Source: CAD feature listing. Evaluate the final solid. Frame: model axes, mm. Face numbers are marked on the shaded views. A direction names the side the tool comes from. Give positions to 0.01 mm unless a question says otherwise; leave off trailing zeros. Order: outer loops, then holes, each group sorted by start corner. A loop starts at its lowest first (then second) coordinate and runs counter-clockwise, first axis right, second up. Notation, with made-up numbers: M 61.5,18 L 96.5,18 A18 ccw 96.5,38 Z; hole C -7,23 d1. An arc over 180 degrees is marked long. Return JSON: item names as keys, results as strings.
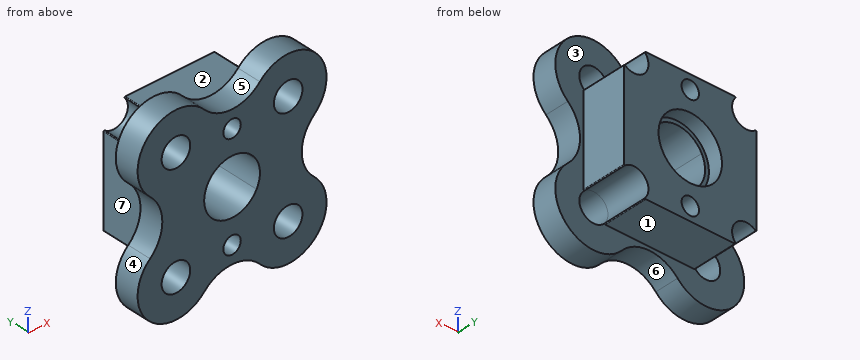
from build123d import *
from build123d.topology import SkipClean

# Parameters (mm, degrees)
SKETCH1_R               = 1.25
BOSS_EXTRUDE1_DEPTH     = 3.5
SKETCH3_R               = 2.05
CUT_EXTRUDE3_DEPTH      = 20.479604719
BOSS_EXTRUDE2_START     = 6.5
SKETCH6_R               = 1.25
BOSS_EXTRUDE2_DEPTH     = 6.5
CUT_EXTRUDE8_DEPTH      = 22.614925399
CUT_EXTRUDE7_DEPTH      = 22.614925399
CUT_EXTRUDE7_DEPTH_BACK = 22.614925399
SKETCH9_R               = 4
SKETCH11_R              = 4.55
CUT_EXTRUDE9_DEPTH      = 2.1
FILLET5_R               = 0.1


with BuildPart() as part:
    # Sketch1 → Boss-Extrude1 (new body)
    with BuildSketch(Plane(origin=(0, 0, 0), x_dir=(1, 0, 0), z_dir=(0, 1, 0))):
        with BuildLine():
            ThreePointArc((3.988860539, -11.759062722), (11.939087297, -11.939087297), (11.759062722, -3.988860539))
            ThreePointArc((11.759062722, -3.988860539), (10, 0), (11.759062722, 3.988860539))
            ThreePointArc((11.759062722, 3.988860539), (11.939087297, 11.939087297), (3.988860539, 11.759062722))
            ThreePointArc((3.988860539, 11.759062722), (0, 10), (-3.988860539, 11.759062722))
            ThreePointArc((-3.988860539, 11.759062722), (-11.939087297, 11.939087297), (-11.759062722, 3.988860539))
            ThreePointArc((-11.759062722, 3.988860539), (-10, 0), (-11.759062722, -3.988860539))
            ThreePointArc((-11.759062722, -3.988860539), (-11.939087297, -11.939087297), (-3.988860539, -11.759062722))
            ThreePointArc((-3.988860539, -11.759062722), (0, -10), (3.988860539, -11.759062722))
        make_face()
        with Locations(Location((0, -7.5, 0), (0, 0, 270))):
            Circle(SKETCH1_R, mode=Mode.SUBTRACT)
        with Locations(Location((0, 7.5, 0), (0, 0, 90))):
            Circle(SKETCH1_R, mode=Mode.SUBTRACT)
    extrude(amount=BOSS_EXTRUDE1_DEPTH)

    # Sketch3 → Cut-Extrude3 (cut, through all)
    with BuildSketch(Plane(origin=(0, 3.5, 0), x_dir=(1, 0, 0), z_dir=(0, 1, 0))):
        with Locations(Location((-8.05, 8.05, 0), (0, 0, 270))):
            Circle(SKETCH3_R)
        with Locations(Location((8.05, 8.05, 0), (0, 0, 270))):
            Circle(SKETCH3_R)
        with Locations(Location((8.05, -8.05, 0), (0, 0, 270))):
            Circle(SKETCH3_R)
        with Locations(Location((-8.05, -8.05, 0), (0, 0, 270))):
            Circle(SKETCH3_R)
    extrude(amount=-CUT_EXTRUDE3_DEPTH, mode=Mode.SUBTRACT)

    # Sketch6 → Boss-Extrude2 (add)
    with SkipClean():  # the faces are left unmerged after this step: merging them gives an invalid solid
        with BuildSketch(Plane(origin=(0, 3.5, 0), x_dir=(1, 0, 0), z_dir=(0, 1, 0)).offset(BOSS_EXTRUDE2_START)):
            with BuildLine():
                Line((6.600862325, 9.5), (-6.600862325, 9.5))
                ThreePointArc((-6.600862325, 9.5), (-6.600431099, 6.600431099), (-9.5, 6.600862325))
                Line((-9.5, 6.600862325), (-9.5, -6.600862325))
                ThreePointArc((-9.5, -6.600862325), (-6.600431099, -6.600431099), (-6.600862325, -9.5))
                Line((-6.600862325, -9.5), (6.600862325, -9.5))
                ThreePointArc((6.600862325, -9.5), (6.600431099, -6.600431099), (9.5, -6.600862325))
                Line((9.5, -6.600862325), (9.5, 6.600862325))
                ThreePointArc((9.5, 6.600862325), (6.600431099, 6.600431099), (6.600862325, 9.5))
            make_face()
            with Locations(Location((0, -7.5, 0), (0, 0, 270))):
                Circle(SKETCH6_R, mode=Mode.SUBTRACT)
            with Locations(Location((0, 7.5, 0), (0, 0, 90))):
                Circle(SKETCH6_R, mode=Mode.SUBTRACT)
        extrude(amount=-BOSS_EXTRUDE2_DEPTH)

    # Sketch10 → Cut-Extrude8 (cut, through all)
    with SkipClean():  # the faces are left unmerged after this step: merging them gives an invalid solid
        with BuildSketch(Plane(origin=(0, 10, 0), x_dir=(1, 0, 0), z_dir=(0, 1, 0))):
            with BuildLine():
                Line((-3.519943181, 1.9), (-3.519943181, -1.9))
                ThreePointArc((-3.519943181, -1.9), (0, -4), (3.519943181, -1.9))
                Line((3.519943181, -1.9), (3.519943181, 1.9))
                ThreePointArc((3.519943181, 1.9), (0, 4), (-3.519943181, 1.9))
            make_face()
        extrude(amount=-CUT_EXTRUDE8_DEPTH, mode=Mode.SUBTRACT)

    # Sketch9 → Cut-Extrude7 (cut, two sides: drawn at the far end of the back side and taken through both)
    with SkipClean():  # the faces are left unmerged after this step: merging them gives an invalid solid
        with BuildSketch(Plane(origin=(0, 10, 0), x_dir=(1, 0, 0), z_dir=(0, 1, 0)).offset(-CUT_EXTRUDE7_DEPTH_BACK)):
            with Locations(Location((0, 0, 0), (0, 0, 90))):
                Circle(SKETCH9_R)
        extrude(amount=CUT_EXTRUDE7_DEPTH + CUT_EXTRUDE7_DEPTH_BACK, mode=Mode.SUBTRACT)

    # Sketch11 → Cut-Extrude9 (cut)
    with SkipClean():  # the faces are left unmerged after this step: merging them gives an invalid solid
        with BuildSketch(Plane(origin=(0, 10, 0), x_dir=(1, 0, 0), z_dir=(0, 1, 0))):
            with Locations(Location((0, 0, 0), (0, 0, 270))):
                Circle(SKETCH11_R)
        extrude(amount=-CUT_EXTRUDE9_DEPTH, mode=Mode.SUBTRACT)

    # Fillet5
    fillet5_edges = [part.edges().sort_by_distance(p)[0] for p in [
        (9.5, 6.75, -6.600862325),
        (6.600862325, 6.75, -9.5),
        (9.5, 6.75, 6.600862325),
        (6.600862325, 6.75, 9.5),
        (-6.600862325, 6.75, 9.5),
        (-9.5, 6.75, 6.600862325),
        (-9.5, 6.75, -6.600862325),
        (-6.600862325, 6.75, -9.5),
    ]]
    fillet(fillet5_edges, radius=FILLET5_R)


solid = part.part
1. Section query D-D (z = -8.05). Return loops of the section in (x, y).
Evaluation:
{"outline": "M -13.55,0 L -10.1,0 L -10.1,3.5 L -13.55,3.5 Z; M -6,0 L -1.12,0 L -1.12,10 L -6,10 Z; M 1.12,0 L 6,0 L 6,10 L 1.12,10 Z; M 10.1,0 L 13.55,0 L 13.55,3.5 L 10.1,3.5 Z"}
2. First-contact query: pin 1 (5 mm diameter, centred on y = 7.5, z = 1, fed in from -X); pin 2 (2 mm diameter, centred on x = 4, y = 3.5, fed in from -Z); pin 3 (2 mm diameter, centred on x = 2, y = 6.5, fed in from +Z); pin 4 (2 mm diameter, centred on x = 0, z = -7.5, fed in from -Y). Flat tips, straight axial feed; report the tip coordinate or a pass-through.
Evaluation:
{"pin 1": "stops at x = -9.5", "pin 2": "stops at z = -12.63", "pin 3": "stops at z = 9.5", "pin 4": "passes through"}
3. Ray query, probe 1 along Z at (x, y) = (8.05, 2.2); probe 2 along X at (y, z) = (9.35, 0); probe 3 along Z at (x, y) = (8.75, 3). Return the intervals inside material, ascending.
Evaluation:
{"probe 1": "z = -13.55 to -10.1, -6 to 6, 10.1 to 13.55", "probe 2": "x = -9.5 to -4.55, 4.55 to 9.5", "probe 3": "z = -13.51 to -9.98, -6.12 to 6.12, 9.98 to 13.51"}
4. Section query C-C (y = 2). Return loops of the section in (x, z).
Evaluation:
{"outline": "M -11.76,-3.99 A5.5 ccw long -3.99,-11.76 A5.4 cw 3.99,-11.76 A5.5 ccw long 11.76,-3.99 A5.4 cw 11.76,3.99 A5.5 ccw long 3.99,11.76 A5.4 cw -3.99,11.76 A5.5 ccw long -11.76,3.99 A5.4 cw Z; hole C -8.05,-8.05 d4.1; hole C -8.05,8.05 d4.1; hole C 0,0 d8; hole C 0,-7.5 d2.5; hole C 0,7.5 d2.5; hole C 8.05,-8.05 d4.1; hole C 8.05,8.05 d4.1"}
5. Section query A-A (z = 0). Return loops of the section in (x, y).
Evaluation:
{"outline": "M -10,0 L -4,0 L -4,7.9 L -4.55,7.9 L -4.55,10 L -9.5,10 L -9.5,3.5 L -10,3.5 Z; M 4,0 L 10,0 L 10,3.5 L 9.5,3.5 L 9.5,10 L 4.55,10 L 4.55,7.9 L 4,7.9 Z"}
6. Set-up query: the marked faces 1, 2 and 3. Return all of +Z, -Z, +X, -X, +Y, -Y with unobstructed straight access to the full face (end or side cutting, diameter ignored); none if empty.
Evaluation:
{"face 1": "-Z, +X, -X, +Y", "face 2": "+Z, +X, -X, +Y", "face 3": "+Y"}
7. Draft query along Z for the marked faces 4, 5, 6 and 7. Return one class per face: pulls with the +Z half, pulls with the -Z half, needs draft (parallel to the pull), parting line crosses it, or undercut.
Evaluation:
{"face 4": "undercut", "face 5": "pulls with the +Z half", "face 6": "pulls with the -Z half", "face 7": "needs draft"}
8. Section query B-B (x = -8.05). Return loops of the section in (y, z).
Evaluation:
{"outline": "M 0,-13.55 L 3.5,-13.55 L 3.5,-10.1 L 0,-10.1 Z; M 0,-6 L 10,-6 L 10,6 L 0,6 Z; M 0,10.1 L 3.5,10.1 L 3.5,13.55 L 0,13.55 Z"}
